```python
from build123d import *

# Parameters (mm, degrees)
SKETCH_1_R          = 10
SKETCH_1_R_2        = 9
M4X0_71_D           = 3.3
M4X0_71_CSINK_D     = 4.05
M4X0_71_CSINK_ANGLE = 90


with BuildPart() as part:
    # По траектории2: sweep along a path in Эскиз2
    with BuildLine(Plane.XY) as sweep_2_path:
        Line((0, 0), (0, 78.426510273))
        Line((0, 78.426510273), (7.471377296, 96.690895762))
    # Эскиз1 → По траектории2 (sweep)
    with BuildSketch(Plane(origin=(0, 0, 0), x_dir=(1, 0, 0), z_dir=(0, 1, 0))):
        Circle(SKETCH_1_R)
        Circle(SKETCH_1_R_2, mode=Mode.SUBTRACT)
    sweep(path=sweep_2_path.line, transition=Transition.RIGHT)

    # Отверстие обработанное метчиком M4x0.71 (through all)
    with Locations(Plane(origin=(8.205564009, 91.642912959, 9.658566578), x_dir=(0.970537064, 0, -0.240951879), z_dir=(0.23978989, -0.098090393, 0.965856658))):
        with Locations((0, 0)):
            CounterSinkHole(M4X0_71_D / 2, M4X0_71_CSINK_D / 2, counter_sink_angle=M4X0_71_CSINK_ANGLE)


solid = part.part
```
Here's how the part is built. I have some questions about the finished solid (model axes, mm). A direction names the side the tool comes from. Coordinates: 2 decimals unless noted, no trailing zeros. Order: outer loops, then holes, each group sorted by start corner. A loop starts at its lowest first (then second) coordinate and runs counter-clockwise, first axis right, second up. Notation, with made-up numbers: (59, 39.5) - (103, 39.5) arc R29 cw to (103, 61.5) - close; hole circle Ø4 at (76.5, 69.5). An arc over 180 degrees is marked (long way). One line per question, with ' | ' between items. Start each with the question number.
1. Please list where these lines run through material, in increasing order: line 1 along X through (y, z) = (23.5, 0); line 2 along Z through (x, y) = (4.5, 72.5). Write a range as [from, to].
2. If we section it at A-A (z = 2.5): Write out the boundary of the cut face in (x, y).
3. If we mould it in two halves opening along Z, with no side actions, what happens to faces 3 (the cylindrical face through (4.75, 94.66, -9.3)), 4 (the flat face through (2, 0, -9)), 5 (the cylindrical face through (-5.826, 90.572, -0.44))? For each: released by +Z, released by -Z, zero draft, split by the parting line, or undercut.
4. Which directions (+Z, -Z, +X, -X, +Y, -Y) give clear straight access to the entire face, cutting with the end or side of a thin tool? Please do faces 1 (the cylindrical face through (9.623, 91.791, 8.525)), 2 (the cylindrical face through (9.54, 40.76, -3)).
5. If we section it at C-C (x = 3.5): Give the number of separate pieces and of enclosed holes in the cut face, and give its area (3 significant figures).
6. If we section it at B-B (y = 31): Write out the boundary of the cut face in (x, z).
7. I'm going to push flat-ended pins straight in: pin 1 Ø6 at (y, z) = (83.5, 6) entering from -X; pin 2 Ø2 at (y, z) = (34.5, 5.5) entering from +X; pin 3 Ø4 at (x, y) = (5.5, 70.5) entering from +Z. Where does each tip first touch, or does it pass through?
8. If we section it at D-D (z = -6): Write out the boundary of the cut face in (x, y), and give its area (3 significant figures).
Model answer:
1) line 1: x = [-10, -9], [9, 10] | line 2: z = [-8.93, -7.79], [7.79, 8.93]
2) outline: (-9.68, 0) - (-8.65, 0) - (-8.65, 80.13) - (-0.53, 99.96) - (-1.49, 100.36) - (-9.68, 80.33) - close; (8.65, 0) - (9.68, 0) - (9.68, 76.52) - (16.43, 93.02) - (15.47, 93.42) - (8.65, 76.73) - close
3) face 3: undercut | face 4: zero draft | face 5: split by the parting line
4) face 1: none | face 2: -Y
5) separate pieces: 3 | enclosed holes: 0 | area: 206 mm²
6) outline: circle Ø20 at (0, 0); hole circle Ø18 at (0, 0)
7) pin 1: stops at x = -8.75 | pin 2: stops at x = 8.93 | pin 3: stops at z = 9.37
8) outline: (-8, 0) - (-6.71, 0) - (-6.71, 79.75) - (1.26, 99.23) - (0.07, 99.72) - (-8, 80) - close; (6.71, 0) - (8, 0) - (8, 76.85) - (14.88, 93.66) - (13.68, 94.15) - (6.71, 77.11) - close | area: 254 mm²
